Here's how the part is built. I have some questions about the finished solid (model axes, mm). Round coordinates to 2 decimals unless told otherwise and drop trailing zeros.
```python
from build123d import *

# Parameters (mm, degrees)
F0_R     = 2.09999979
F1_DEPTH = 1000


# Not quite as in the source:
# - ends of sketch curves that miss each other by under 0.0002 mm in the source are joined


with BuildPart() as f1:
    # F0 (on Top) → F1 (new body)
    with BuildSketch(Plane.XY):
        with BuildLine():
            Line((-4.639999536, 10), (-8.50000015, 10))
            ThreePointArc((-8.50000015, 10), (-9.5606602157, 9.5606602157), (-10, 8.50000015))
            Line((-10, 8.50000015), (-10, 4.639999536))
            Line((-10, 4.639999536), (-8.19999818, 2.839999716))
            Line((-8.19999818, 2.839999716), (-8.19999818, 5.4993384501))
            Line((-8.19999818, 5.4993384501), (-6.559999344, 5.4993384501))
            Line((-6.559999344, 5.4993384501), (-3.9006596099, 2.839999716))
            Line((-3.9006596099, 2.839999716), (-3.9006596099, 0.19999898))
            Line((-3.9006596099, 0.19999898), (-3.7006596299, -1e-06))
            Line((-3.7006596299, -1e-06), (-3.9006596099, -0.20000098))
            Line((-3.9006596099, -0.20000098), (-3.9006596099, -2.840000716))
            Line((-3.9006596099, -2.840000716), (-6.559999344, -5.4993404501))
            Line((-6.559999344, -5.4993404501), (-8.19999818, -5.4993404501))
            Line((-8.19999818, -5.4993404501), (-8.19999818, -2.840000716))
            Line((-8.19999818, -2.840000716), (-10, -4.640000536))
            Line((-10, -4.640000536), (-10, -8.50000115))
            ThreePointArc((-10, -8.50000115), (-9.5606602157, -9.5606612157), (-8.50000015, -10.000001))
            Line((-8.50000015, -10.000001), (-4.639999536, -10))
            Line((-4.639999536, -10), (-2.839999716, -8.20000018))
            Line((-2.839999716, -8.20000018), (-5.4993394501, -8.20000018))
            Line((-5.4993394501, -8.20000018), (-5.4993394501, -6.560000344))
            Line((-5.4993394501, -6.560000344), (-2.839999716, -3.9006606099))
            Line((-2.839999716, -3.9006606099), (-0.19999898, -3.9006606099))
            Line((-0.19999898, -3.9006606099), (1e-06, -3.7006606299))
            Line((1e-06, -3.7006606299), (0.20000098, -3.9006606099))
            Line((0.20000098, -3.9006606099), (2.839999716, -3.9006606099))
            Line((2.839999716, -3.9006606099), (5.4993414501, -6.560000344))
            Line((5.4993414501, -6.560000344), (5.4993414501, -8.20000018))
            Line((5.4993414501, -8.20000018), (2.839999716, -8.20000018))
            Line((2.839999716, -8.20000018), (4.639999536, -10))
            Line((4.639999536, -10), (8.50000015, -10))
            ThreePointArc((8.50000015, -10), (9.5606602157, -9.5606612157), (10, -8.50000115))
            Line((10, -8.50000115), (10, -4.640000536))
            Line((10, -4.640000536), (8.20000018, -2.840000716))
            Line((8.20000018, -2.840000716), (8.20000018, -5.4993404501))
            Line((8.20000018, -5.4993404501), (6.560000344, -5.4993404501))
            Line((6.560000344, -5.4993404501), (3.9006596099, -2.840000716))
            Line((3.9006596099, -2.840000716), (3.9006596099, -0.20000098))
            Line((3.9006596099, -0.20000098), (3.7006596299, -1e-06))
            Line((3.7006596299, -1e-06), (3.9006596099, 0.19999898))
            Line((3.9006596099, 0.19999898), (3.9006596099, 2.839999716))
            Line((3.9006596099, 2.839999716), (6.560000344, 5.4993384501))
            Line((6.560000344, 5.4993384501), (8.20000018, 5.4993384501))
            Line((8.20000018, 5.4993384501), (8.20000018, 2.839999716))
            Line((8.20000018, 2.839999716), (10, 4.639999536))
            Line((10, 4.639999536), (10, 8.50000015))
            ThreePointArc((10, 8.50000015), (9.5606602157, 9.5606602157), (8.50000015, 10))
            Line((8.50000015, 10), (4.639999536, 10))
            Line((4.639999536, 10), (2.839999716, 8.20000018))
            Line((2.839999716, 8.20000018), (5.4993414501, 8.20000018))
            Line((5.4993414501, 8.20000018), (5.4993414501, 6.559998344))
            Line((5.4993414501, 6.559998344), (2.839999716, 3.9006596099))
            Line((2.839999716, 3.9006596099), (0.20000098, 3.9006596099))
            Line((0.20000098, 3.9006596099), (1e-06, 3.7006596299))
            Line((1e-06, 3.7006596299), (-0.19999898, 3.9006596099))
            Line((-0.19999898, 3.9006596099), (-2.839999716, 3.9006596099))
            Line((-2.839999716, 3.9006596099), (-5.4993394501, 6.559998344))
            Line((-5.4993394501, 6.559998344), (-5.4993394501, 8.20000018))
            Line((-5.4993394501, 8.20000018), (-2.839999716, 8.20000018))
            Line((-2.839999716, 8.20000018), (-4.639999536, 10))
        make_face()
        Polygon((-6.5693393431, -8.20000018), (-8.19999818, -8.20000018), (-8.19999818, -6.5693403431), (-7.629998237, -6.5693403431), (-6.5693393431, -7.630000237), align=None, mode=Mode.SUBTRACT)
        Polygon((8.20000018, -8.20000018), (6.5693393431, -8.20000018), (6.5693393431, -7.630000237), (7.630002237, -6.5693403431), (8.20000018, -6.5693403431), align=None, mode=Mode.SUBTRACT)
        with Locations((1e-06, -1e-06)):
            Circle(F0_R, mode=Mode.SUBTRACT)
        Polygon((-8.19999818, 8.20000018), (-6.5693393431, 8.20000018), (-6.5693393431, 7.629999237), (-7.629998237, 6.5693393431), (-8.19999818, 6.5693393431), align=None, mode=Mode.SUBTRACT)
        Polygon((6.5693393431, 8.20000018), (8.20000018, 8.20000018), (8.20000018, 6.5693393431), (7.630002237, 6.5693393431), (6.5693393431, 7.629999237), align=None, mode=Mode.SUBTRACT)
    extrude(amount=F1_DEPTH)


solid = f1.part
```
1. I need wall thicknesses on probe 1 along Y at (x, z) = (-7.75, 950); probe 2 along Y at (x, z) = (6.5, 613); probe 3 along X at (y, z) = (-3.5, 244.5). Which ranges of each line are inside material? Lowest first, please.
Evaluation:
probe 1: y = -10 to -8.2, -6.57 to -5.5, 5.5 to 6.57, 8.2 to 10
probe 2: y = -10 to -5.44, 5.44 to 10
probe 3: x = -8.86 to -8.2, -4.56 to 4.56, 8.2 to 8.86
2. I'm going to push flat-ended pins straight in: P1, Ø2, axis at y = 3, z = 130.5, coming from the -X side; P2, Ø1.5, axis at y = 2, z = 395.5, coming from the +X side. Where does each tip first touch, or does it pass through?
Evaluation:
P1: stops at x = -9.36
P2: stops at x = 3.9
3. If we section it at A-A, the plane z = 300.5: State how many separate pieces and enclosed holes the cut face has, and give its area (3 significant figures).
Evaluation:
separate pieces: 1
enclosed holes: 5
area: 161 mm2
